from build123d import *

# Parameters (mm, degrees)
SKETCH1_R           = 1.5825
SKETCH1_W           = 10
SKETCH1_H           = 12.5
BOSS_EXTRUDE1_DEPTH = 2.5
SKETCH2_W           = 5.2
SKETCH2_H           = 16
BOSS_EXTRUDE2_DEPTH = 2.5
SKETCH3_W           = 1.7
SKETCH3_H           = 4.72
CUT_EXTRUDE1_DEPTH  = 30.1317696
BOSS_EXTRUDE3_DEPTH = 3.5
BOSS_EXTRUDE5_DEPTH = 3.5
SKETCH10_R          = 4
BOSS_EXTRUDE6_DEPTH = 1.875
SKETCH11_R          = 1.585
CUT_EXTRUDE4_DEPTH  = 30.669560778
SKETCH12_R          = 4
CUT_EXTRUDE5_DEPTH  = 1
FILLET1_R           = 1
FILLET2_R           = 1
SKETCH14_W          = 11.670795551
SKETCH14_H          = 6
BOSS_EXTRUDE7_DEPTH = 2
SKETCH6_R           = 1.475
CUT_EXTRUDE3_DEPTH  = 16.7
CUT_EXTRUDE8_DEPTH  = 1.7
FILLET3_R           = 2
FILLET4_R           = 0.05


with BuildPart() as part:
    # Sketch1 → Boss-Extrude1 (new body)
    # profile 1 of 2: a face of its own
    with BuildSketch(Plane.XY):
        with BuildLine():
            ThreePointArc((0, 6.25), (-6.25, 0), (0, -6.25))
            Line((0, -6.25), (12.7, -6.25))
            Line((12.7, -6.25), (12.7, 6.25))
            Line((12.7, 6.25), (0, 6.25))
        make_face()
        Circle(SKETCH1_R, mode=Mode.SUBTRACT)
    # profile 2 of 2: a face of its own
    with BuildSketch(Plane.XY):
        with Locations((17.7, 0)):
            Rectangle(SKETCH1_W, SKETCH1_H)
    extrude(amount=BOSS_EXTRUDE1_DEPTH)

    # Sketch2 → Boss-Extrude2 (add)
    with BuildSketch(Plane.XY.offset(2.5)):
        with Locations((25.3, 0)):
            Rectangle(SKETCH2_W, SKETCH2_H)
    extrude(amount=-BOSS_EXTRUDE2_DEPTH)

    # Sketch3 → Cut-Extrude1 (cut, through all)
    with BuildSketch(Plane.XY.offset(2.5)):
        with Locations((21.85, 0)):
            Rectangle(SKETCH3_W, SKETCH3_H)
    extrude(amount=-CUT_EXTRUDE1_DEPTH, mode=Mode.SUBTRACT)


with BuildPart() as body_2:
    # Sketch7 → Boss-Extrude3 (new body)
    with BuildSketch(Plane.XZ.offset(6.25)):
        with BuildLine():
            Line((6.129900512, 3.210673711), (6.129900512, 4.710673711))
            ThreePointArc((6.129900512, 4.710673711), (6.694341527, 4.327552018), (7.360579964, 4.180915603))
            ThreePointArc((7.360579964, 4.180915603), (7.789326283, 4.199870579), (8.206709695, 4.299739418))
            ThreePointArc((8.206709695, 4.299739418), (15.494742209, 6.151071465), (22.7, 4))
            Line((22.7, 4), (22.7, 2.5))
            ThreePointArc((22.7, 2.5), (15.494742209, 4.651071465), (8.206709695, 2.799739418))
            ThreePointArc((8.206709695, 2.799739418), (7.789326283, 2.699870579), (7.360579964, 2.680915603))
            ThreePointArc((7.360579964, 2.680915603), (6.694341527, 2.827552018), (6.129900512, 3.210673711))
        make_face()
    extrude(amount=-BOSS_EXTRUDE3_DEPTH)


with BuildPart() as body_3:
    # Sketch9 → Boss-Extrude5 (new body)
    with BuildSketch(Plane.XZ.offset(6.25)):
        Polygon((22.7, 4), (25.104907101, 2.5), (22.7, 2.5), align=None)
    extrude(amount=-BOSS_EXTRUDE5_DEPTH)

    # Combine1: union body 2
    add(body_2.part)


with BuildPart() as body_3_2:
    # Mirror5: mirrored copy
    add(body_3.part.mirror(Plane(origin=(0, 0, 0), x_dir=(0, 0, 1), z_dir=(0, -1, 0))))


with BuildPart() as part_1:
    add(part.part)

    # Combine4: union body 3, body 3 2
    add(body_3.part)
    add(body_3_2.part)

    # Sketch10 → Boss-Extrude6 (add)
    with BuildSketch(Plane(origin=(0, 0, 0), x_dir=(-1, 0, 0), z_dir=(0, 0, -1))):
        with Locations(Location((0, 0, 0), (0, 0, 180))):
            Circle(SKETCH10_R)
    extrude(amount=BOSS_EXTRUDE6_DEPTH)

    # Sketch11 → Cut-Extrude4 (cut, through all)
    with BuildSketch(Plane.XY):
        Circle(SKETCH11_R)
    extrude(amount=-CUT_EXTRUDE4_DEPTH, mode=Mode.SUBTRACT)

    # Sketch12 → Cut-Extrude5 (cut)
    with BuildSketch(Plane.XY.offset(2.5)):
        Circle(SKETCH12_R)
    extrude(amount=-CUT_EXTRUDE5_DEPTH, mode=Mode.SUBTRACT)

    # Fillet1
    fillet1_edges = [part_1.edges().sort_by_distance(p)[0] for p in [
        (-4, 0, 2.5),
    ]]
    fillet(fillet1_edges, radius=FILLET1_R - 0.0001)  # a hair under: the kernel refuses the full size

    # Fillet2
    fillet2_edges = [part_1.edges().sort_by_distance(p)[0] for p in [
        (-4, 0, -1.875),
    ]]
    fillet(fillet2_edges, radius=FILLET2_R)

    # Sketch14 → Boss-Extrude7 (add)
    with BuildSketch(Plane(origin=(0, 0, 0), x_dir=(-1, 0, 0), z_dir=(0, 0, -1))):
        with Locations((-22.064602224, 0)):
            Rectangle(SKETCH14_W, SKETCH14_H)
    extrude(amount=BOSS_EXTRUDE7_DEPTH)

    # Sketch6 → Cut-Extrude3 (cut)
    with BuildSketch(Plane(origin=(27.9, 0, 0), x_dir=(0, 0, -1), z_dir=(1, 0, 0))):
        with Locations((-1.25, 0)):
            Circle(SKETCH6_R)
    extrude(amount=-CUT_EXTRUDE3_DEPTH, mode=Mode.SUBTRACT)

    # Sketch16 → Cut-Extrude8 (cut)
    with BuildSketch(Plane(origin=(21, 0, 0), x_dir=(0, 0, -1), z_dir=(1, 0, 0))):
        Polygon((1.475093271, 0), (0.112546635, 2.36), (-2.612546635, 2.36), (-3.975093271, 0), (-2.612546635, -2.36), (0.112546635, -2.36), align=None)
    extrude(amount=CUT_EXTRUDE8_DEPTH, mode=Mode.SUBTRACT)

    # Fillet3
    fillet3_edges = [part_1.edges().sort_by_distance(p)[0] for p in [
        (22.064602225, -3, 0),
        (22.064602225, 3, 0),
    ]]
    fillet(fillet3_edges, radius=FILLET3_R - 0.0001)  # a hair under: the kernel refuses the full size

    # Fillet4
    fillet4_edges = [part_1.edges().sort_by_distance(p)[0] for p in [
        (16.1, -0.783022988, 2.5),
        (25.3, -0.783022988, 2.5),
        (25.3, 0.783022988, 2.5),
        (16.1, 0.783022988, 2.5),
        (13.714602225, -0.783022988, 0),
        (13.714602225, 0.783022988, 0),
    ]]
    fillet(fillet4_edges, radius=FILLET4_R)


solid = part_1.part
Check sheet for the modelled part. Datum: model origin and axes. Units: mm. A direction names the side the tool comes from. Coordinates: 2 decimals unless noted, no trailing zeros. Loops run counter-clockwise (first coordinate to the right, second up) from the corner with the lowest first, then second, coordinate; pieces in that order, holes last. Notation, with made-up numbers: (1.5, 85.25) -> (33.5, 85.25) arc R23 ccw to (33.5, 110.25) -> close; hole circle Ø8 at (23.25, -14). An arc over 180 degrees is marked (long way). Answer in a Markdown table with one row per item.
1. Go/stop test with flat-tipped pins: pin 1 (1.8 mm diameter, centred on x = 11.5, z = 5, fed in from +Y); pin 2 (1.1 mm diameter, centred on x = 12.5, z = 3.5, fed in from -Y); pin 3 (0.8 mm diameter, centred on x = 16.5, z = 1.5, fed in from -Y); pin 4 (5 mm diameter, centred on x = 8, y = 1.5, fed in from -Z). Record where each tip stops, or that it passes through.
Check values:
| item | result |
|---|---|
| pin 1 | stops at y = 6.25 |
| pin 2 | passes through |
| pin 3 | stops at y = -6.25 |
| pin 4 | stops at z = 0 |
2. Sectioned sample at B-B, the plane x = 14. Record the boundary of the cut face in (y, z) (3 decimals).
Check values:
| item | result |
|---|---|
| outline | (-6.25, 0) -> (-0.941, 0) arc R0.05 ccw to (-0.91, 0.089) arc R1.475 cw to (-0.91, 2.411) arc R0.05 ccw to (-0.941, 2.5) -> (-6.25, 2.5) -> close; (-6.25, 4.603) -> (-2.75, 4.603) -> (-2.75, 6.103) -> (-6.25, 6.103) -> close; (0.91, 0.089) arc R0.05 ccw to (0.941, 0) -> (6.25, 0) -> (6.25, 2.5) -> (0.941, 2.5) arc R0.05 ccw to (0.91, 2.411) arc R1.475 cw to start; (2.75, 4.603) -> (6.25, 4.603) -> (6.25, 6.103) -> (2.75, 6.103) -> close |
3. Material ranges on line 1 along Y through (x, z) = (15.75, 1.25) (3 decimals); line 2 along X through (y, z) = (0, 1.15); line 3 along Y through (x, z) = (0, -0.75) (3 decimals), recorded low to high. Write a range as [from, to].
Check values:
| item | result |
|---|---|
| line 1 | y = [-6.25, -1.475], [1.475, 6.25] |
| line 2 | x = [-6.25, -1.58], [1.58, 11.2] |
| line 3 | y = [-4, -1.585], [1.585, 4] |
4. Access from +Z, -Z, +X, -X, +Y, -Y to the whole of each face (thin tool, end or side, straight path). Record for faces 5 (the face through (21, -0.6, -0.3)), 6 (the face through (22.7, -7, 1)), 7 (the face through (16, -2.75, 5)).
Check values:
| item | result |
|---|---|
| face 5 | +Z |
| face 6 | +Z, -Z, -X, -Y |
| face 7 | +Z, +X, -X |
5. Sectioned sample at A-A, the plane x = 21.5. Give the number of separate pieces and of enclosed holes in the cut face, then the cut area to 3 significant figures.
Check values:
| item | result |
|---|---|
| separate pieces | 3 |
| enclosed holes | 0 |
| area | 39.9 mm2 |
6. Sectioned sample at C-C, the plane y = 5.5. Record the boundary of the cut face in (x, z).
Check values:
| item | result |
|---|---|
| outline | (-2.97, 0) -> (27.9, 0) -> (27.9, 2.5) -> (25.1, 2.5) -> (22.7, 4) arc R14.12 ccw to (8.21, 4.3) arc R2.25 cw to (7.36, 4.18) arc R1.81 cw to (6.13, 4.71) -> (6.13, 3.21) arc R1.81 ccw to (7.36, 2.68) arc R2.25 ccw to (8.21, 2.8) arc R14.12 cw to (22.7, 2.5) -> (-2.97, 2.5) -> close |
7. Release check for a two-part mould opening along Y. For faces 1 (the face through (22, -2.36, 1)), 2 (the face through (11, -6.25, 1)), 3 (the face through (-6.25, 0.14, 1.23)), 4 (the face through (22.7, 7, 1)) record: released by +Y, released by -Y, zero draft, split by the parting line, or undercut.
Check values:
| item | result |
|---|---|
| face 1 | undercut |
| face 2 | released by -Y |
| face 3 | split by the parting line |
| face 4 | zero draft |
